```python
from build123d import *

# Parameters (mm, degrees)
BOSS_EXTRUDE1_DEPTH      = 25
SKETCH2_R                = 25
BOSS_EXTRUDE2_DEPTH      = 18
BOSS_EXTRUDE3_DEPTH      = 18
BOSS_EXTRUDE4_DEPTH      = 20
BOSS_EXTRUDE4_DEPTH_BACK = 36
SKETCH4_R                = 25
SKETCH5_R                = 18
BOSS_EXTRUDE5_DEPTH      = 18
BOSS_EXTRUDE6_START      = -18
SKETCH6_R                = 18
BOSS_EXTRUDE6_DEPTH      = 18
HOLE1_D                  = 32
HOLE2_D                  = 25
HOLE3_D                  = 15


with BuildPart() as part:
    # Sketch1 → Boss-Extrude1 (new, symmetric)
    with BuildSketch(Plane.XY):
        Polygon((-31, 0), (-17, 0), (-17, 15.39), (17, 15.39), (17, 0), (31, 0), (31, 27.39), (17, 27.39), (17, 110), (-17, 110), (-17, 27.39), (-31, 27.39), align=None)
    extrude(amount=BOSS_EXTRUDE1_DEPTH, both=True)

    # Sketch2 → Boss-Extrude2 (add)
    with BuildSketch(Plane(origin=(-17, 0, 0), x_dir=(0, 0, -1), z_dir=(1, 0, 0))):
        Circle(SKETCH2_R)
    boss_extrude2 = extrude(amount=-BOSS_EXTRUDE2_DEPTH)

    # Mirror1: Boss-Extrude2 across plane
    add(boss_extrude2.mirror(Plane(origin=(0, 0, 0), x_dir=(0, 0, 1), z_dir=(1, 0, 0))))

    # Sketch3 → Boss-Extrude3 (add, symmetric)
    with BuildSketch(Plane(origin=(0, 122.5, 0), x_dir=(1, 0, 0), z_dir=(0, 1, 0))):
        Polygon((-18, 0), (0, 0), (0, -45), (14, -45), (14, -85), (0, -85), (0, -59), (-18, -59), (-18, -85), (-32, -85), (-32, -45), (-18, -45), align=None)
    extrude(amount=BOSS_EXTRUDE3_DEPTH, both=True)

    # Sketch4 → Boss-Extrude4 (add, two sides: drawn at the far end of the back side and taken through both)
    with BuildSketch(Plane(origin=(0, 0, 0), x_dir=(0, 0, -1), z_dir=(1, 0, 0)).offset(-BOSS_EXTRUDE4_DEPTH_BACK)):
        with Locations((0, 115.5)):
            Circle(SKETCH4_R)
    extrude(amount=BOSS_EXTRUDE4_DEPTH + BOSS_EXTRUDE4_DEPTH_BACK)

    # Sketch5 → Boss-Extrude5 (add)
    with BuildSketch(Plane(origin=(0, 0, 0), x_dir=(0, 0, -1), z_dir=(1, 0, 0))):
        with Locations(Location((-85, 122.5, 0), (0, 0, 270))):
            Circle(SKETCH5_R)
    extrude(amount=BOSS_EXTRUDE5_DEPTH)

    # Sketch6 → Boss-Extrude6 (add)
    with BuildSketch(Plane(origin=(-18, 0, 0), x_dir=(0, 0, -1), z_dir=(1, 0, 0)).offset(BOSS_EXTRUDE6_START)):
        with Locations(Location((-85, 122.5, 0), (0, 0, 270))):
            Circle(SKETCH6_R)
    extrude(amount=BOSS_EXTRUDE6_DEPTH)

    # Hole1 (through all)
    with Locations(Plane(origin=(35, 0, 0), x_dir=(0, 0, -1), z_dir=(1, 0, 0))):
        with Locations((0, 0)):
            Hole(HOLE1_D / 2)

    # Hole2 (through all)
    with Locations(Plane(origin=(20, 0, 0), x_dir=(0, 0, -1), z_dir=(1, 0, 0))):
        with Locations((0, 115.5)):
            Hole(HOLE2_D / 2)

    # Hole3 (through all)
    with Locations(Plane(origin=(18, 0, 0), x_dir=(0, 0, -1), z_dir=(1, 0, 0))):
        with Locations((-85, 122.5)):
            Hole(HOLE3_D / 2)


solid = part.part
```
The listing builds one solid part. Answer for the finished solid, in the listing's coordinates (mm). A direction names the side the tool comes from. Give positions to 0.01 mm unless a question says otherwise; leave off trailing zeros. Order: outer loops, then holes, each group sorted by start corner. A loop starts at its lowest first (then second) coordinate and runs counter-clockwise, first axis right, second up. Notation, with made-up numbers: (-16.5, -10) - (29.5, -10) arc R27 cw to (29.5, 25) - close; hole circle Ø7 at (-36, 34.5). An arc over 180 degrees is marked (long way). Answer in a Markdown table with one row per item. Add a question column.
Q1. The part is cut by section B-B (y = 122.5). Give the number of separate pieces and of enclosed holes in the cut face, then the cut area to 3 significant figures.
Q2. Given P1, Ø12, axis at x = 22.5, z = -8, coming from the +Y side; P2, Ø9, axis at x = -6, y = 114, coming from the +Z side; P3, Ø17, axis at y = 122.5, z = 85, coming from the -X side; P4, Ø1, axis at x = 18, y = 25, coming from the +Z side, each flat-ended and moving along its own axis, determine where each tip first touches the part or whether it passes through.
Q3. For a pull along Z with two mould halves and no side action, classify faces 6 (the flat face through (-36, 121.4, 11.5)), 7 (the flat face through (-18, 123, 33)), 8 (the flat face through (-9, 123, 59)) as released by +Z, released by -Z, zero draft, split by the parting line, or undercut.
Q4. The part is cut by section A-A (x = -24.5). Determine the outline of the cut face in (y, z), then the cut area to 3 significant figures.
Q5. The part is cut by section C-C (y = 19). Determine the outline of the cut face in (x, z).
Q6. Which of the six approach directions +Z, -Z, +X, -X, +Y, -Y give full straight-line access (tool end or side, diameter ignored) to faces 1 (the flat face through (20, 121.4, 11.5)), 2 (the flat face through (17, -18, 0)), 3 (the flat face through (-24, 27.39, 0)), 4 (the flat face through (-35, -16.3, 0.3)), 5 (the flat face through (7, 123, 45))?
Q7. Find the intervals of material crossed by line 1 along Z through (x, y) = (-3, 115) (3 decimals); line 2 along Y through (x, z) = (6, 0); line 3 along Z through (x, y) = (-6, 77), in increasing order. Write a range as [from, to].
Q8. The part is cut by section D-D (y = 99.5). Determine the outline of the cut face in (x, z), then the cut area to 3 significant figures.
Determined:
| question | item | result |
|---|---|---|
| 1 | separate pieces | 4 |
| 1 | enclosed holes | 0 |
| 1 | area | 3,530 mm² |
| 2 | P1 | stops at y = 140.37 |
| 2 | P2 | stops at z = 59 |
| 2 | P3 | stops at x = -36 |
| 2 | P4 | stops at z = 25 |
| 3 | face 6 | zero draft |
| 3 | face 7 | undercut |
| 3 | face 8 | released by +Z |
| 4 | outline | (0, -25) - (27.39, -25) - (27.39, 25) - (0, 25) arc R25 ccw to start; circle Ø50 at (115.5, 0); (104.5, 45) - (140.5, 45) - (140.5, 85) arc R18 ccw to (104.5, 85) - close; hole circle Ø32 at (0, 0); hole circle Ø25 at (115.5, 0); hole circle Ø15 at (122.5, 85) |
| 4 | area | 4,790 mm² |
| 5 | outline | (-35, -16.25) - (-31, -16.25) - (-31, -25) - (31, -25) - (31, -16.25) - (35, -16.25) - (35, 16.25) - (31, 16.25) - (31, 25) - (-31, 25) - (-31, 16.25) - (-35, 16.25) - close |
| 6 | face 1 | +Z, -Z, +X, +Y |
| 6 | face 2 | +Z, -Z, -Y |
| 6 | face 3 | +Z, -Z, -X |
| 6 | face 4 | +Z, -Z, -X, -Y |
| 6 | face 5 | +X, +Y, -Y |
| 7 | line 1 | z = [-24.995, -12.49], [12.49, 59] |
| 7 | line 2 | y = [16, 103], [128, 140.5] |
| 7 | line 3 | z = [-25, 25] |
| 8 | outline | (-36, -19.21) - (-17, -19.21) - (-17, -25) - (17, -25) - (17, -19.21) - (20, -19.21) - (20, 19.21) - (17, 19.21) - (17, 25) - (-17, 25) - (-17, 19.21) - (-36, 19.21) - close |
| 8 | area | 2,550 mm² |
